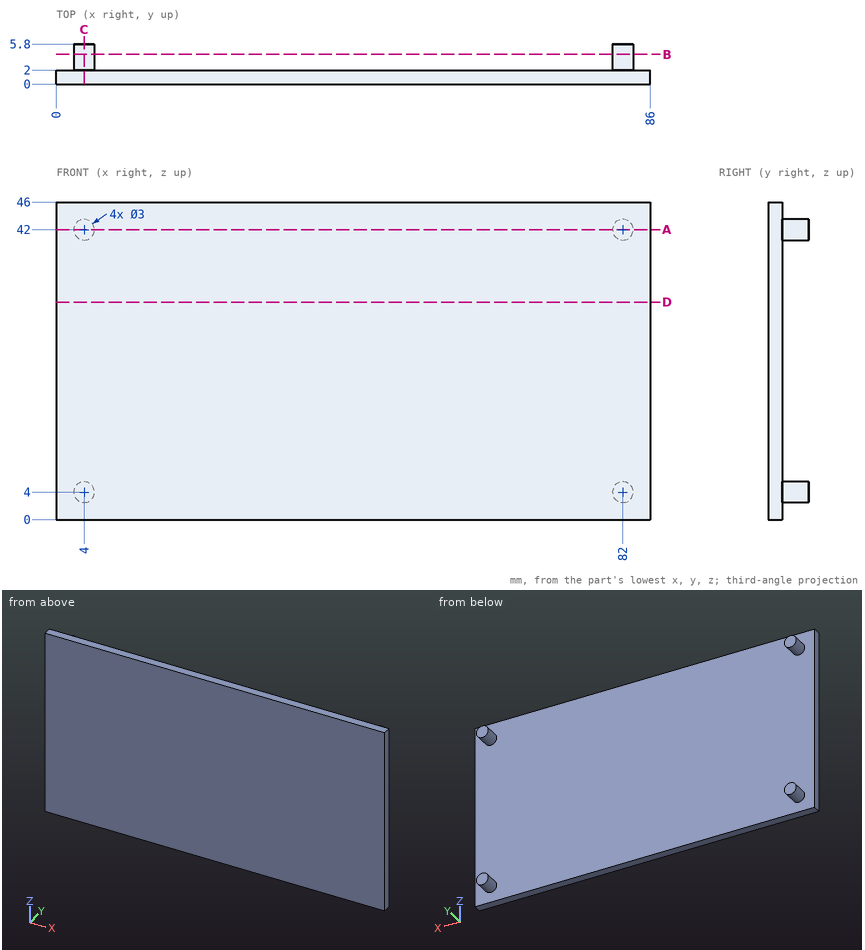
Design review of the part shown in the three views and the two pictorial views. Dimensions are in mm from the part's minimum x, y and z. Round coordinates to 2 decimals unless told otherwise and drop trailing zeros. Write each loop counter-clockwise with the first axis right and the second up, starting at its lowest first coordinate (ties: lowest second). Pieces come first, ordered by that corner, then holes. Notation, with made-up numbers: (-29, 30) - (-18, 30) arc R23 ccw to (-18, 57) - close; hole circle Ø8 at (43, 42.25). An arc over 180 degrees is marked (long way). Answer as CSV lines item,"result". Start each with the question number.
(1) Add section C-C, the plane x = 4. State the section outline as (y, z) points.
(2) For line 1 (Y direction, x = 67.5, z = 29); line 2 (X direction, y = 4.25, z = 41.5); line 3 (Z direction, x = 5, y = 2.7), list the stretches that pass through material, from the lowest coordinate up.
(3) Add section B-B, the plane y = 4.3. State the section outline as (x, z) points.
(4) For pin 1 (23 mm diameter, centred on x = 34.5, z = 22.5, fed in from +Y), flat-tipped, find the tip position at first contact; note if it passes through.
(5) Add section D-D, the plane z = 31.5. State the section outline as (x, y) points, plus the area to 3 significant figures.
(6) Add section A-A, the plane z = 42. State the section outline as (x, y) points, plus the area to 3 significant figures.
From the geometry:
1,outline,"(0, 0) - (2, 0) - (2, 2.5) - (5.8, 2.5) - (5.8, 5.5) - (2, 5.5) - (2, 40.5) - (5.8, 40.5) - (5.8, 43.5) - (2, 43.5) - (2, 46) - (0, 46) - close"
2,line 1,"y = 0 to 2"
2,line 2,"x = 2.59 to 5.41, 80.59 to 83.41"
2,line 3,"z = 2.88 to 5.12, 40.88 to 43.12"
3,outline,"circle Ø3 at (4, 4); circle Ø3 at (4, 42); circle Ø3 at (82, 4); circle Ø3 at (82, 42)"
4,pin 1,"stops at y = 2"
5,outline,"(0, 0) - (86, 0) - (86, 2) - (0, 2) - close"
5,area,"172 mm²"
6,outline,"(0, 0) - (86, 0) - (86, 2) - (83.5, 2) - (83.5, 5.8) - (80.5, 5.8) - (80.5, 2) - (5.5, 2) - (5.5, 5.8) - (2.5, 5.8) - (2.5, 2) - (0, 2) - close"
6,area,"195 mm²"
